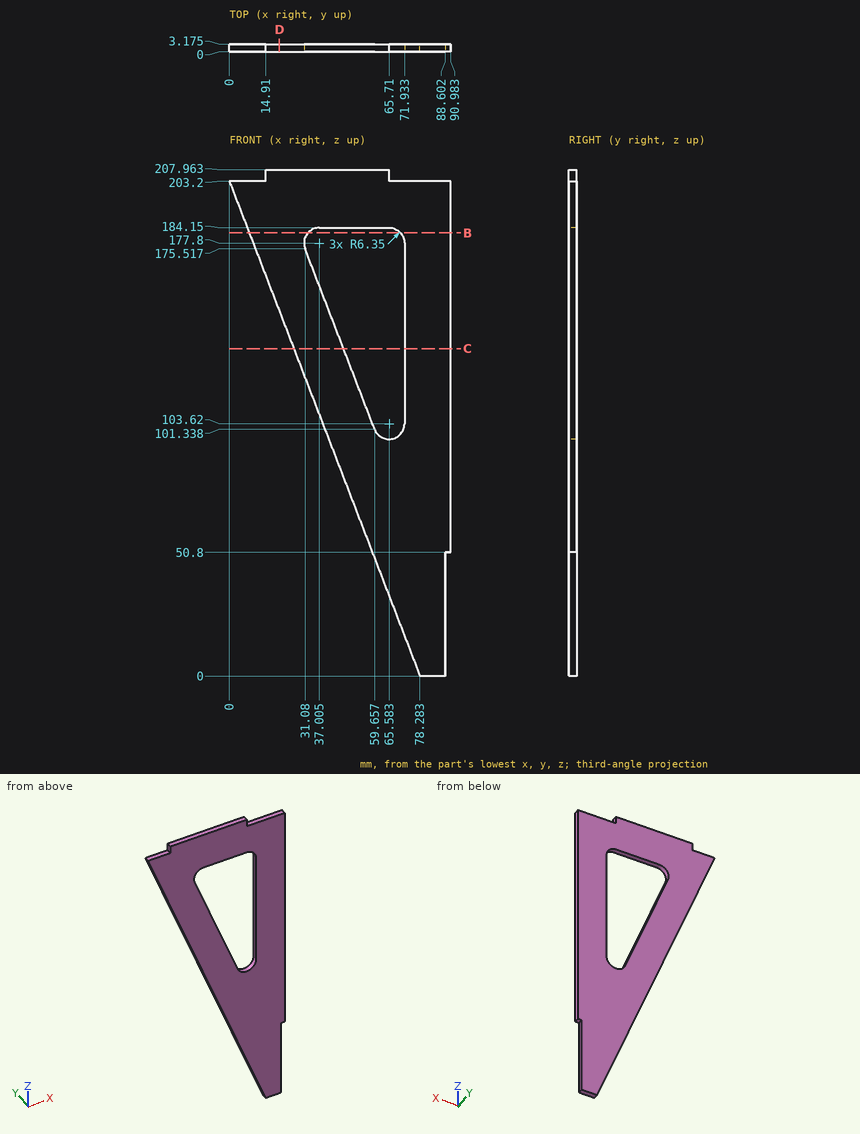
Design review of the part shown in the three views and the two pictorial views. Dimensions are in mm from the part's minimum x, y and z. Give positions to 0.01 mm unless a question says otherwise; leave off trailing zeros. Write each loop counter-clockwise with the first axis right and the second up, starting at its lowest first coordinate (ties: lowest second). Pieces come first, ordered by that corner, then holes. Notation, with made-up numbers: M 77,57 L 130,57 A34 ccw 130,90 Z; hole C -40,-29.5 d5. An arc over 180 degrees is marked long. Answer in a Markdown table with one row per item.
Item 1: For P1, Ø1.9, axis at x = 90, y = 2.5, coming from the -Z side; P2, Ø1, axis at y = 1.5, z = 205.5, coming from the +X side; P3, Ø1, axis at x = 4, y = 1.5, coming from the +Z side, all flat-tipped, find the tip position at first contact; note any pin that passes through.
Check sheet entries:
| item | result |
|---|---|
| P1 | z = 50.8 |
| P2 | x = 65.71 |
| P3 | z = 203.2 |
Item 2: For line 1 along X through (y, z) = (1.55, 136) (1 decimal); line 2 along X through (y, z) = (1.7, 129) (1 decimal); line 3 along X through (y, z) = (0.4, 19.5), list the stretches that pass through material, from the lowest coordinate up.
Check sheet entries:
| item | result |
|---|---|
| line 1 | 25.9 to 46.3, 71.9 to 91 |
| line 2 | 28.6 to 49, 71.9 to 91 |
| line 3 | 70.77 to 88.6 |
Item 3: Add section D-D on x = 20.5. Give the boundary of the cut face in (y, z) (1 decimal), plus the area to 3 significant figures.
Check sheet entries:
| item | result |
|---|---|
| outline | M 0,150 L 3.2,150 L 3.2,208 L 0,208 Z |
| area | 184 mm2 |
Item 4: Add section B-B on z = 182. Give the boundary of the cut face in (x, y) (1 decimal), plus the area to 3 significant figures.
Check sheet entries:
| item | result |
|---|---|
| outline | M 8.2,0 L 32.2,0 L 32.2,3.2 L 8.2,3.2 Z; M 70.3,0 L 91,0 L 91,3.2 L 70.3,3.2 Z |
| area | 142 mm2 |
Item 5: Add section C-C on z = 134.5. Give the boundary of the cut face in (x, y) (1 decimal), plus the area to 3 significant figures.
Check sheet entries:
| item | result |
|---|---|
| outline | M 26.5,0 L 46.9,0 L 46.9,3.2 L 26.5,3.2 Z; M 71.9,0 L 91,0 L 91,3.2 L 71.9,3.2 Z |
| area | 125 mm2 |
